Part model, mm, in its own coordinate system. Face numbers are marked on the shaded views. A direction names the side the tool comes from. Round coordinates to 2 decimals unless told otherwise and drop trailing zeros. Write each loop counter-clockwise with the first axis right and the second up, starting at its lowest first coordinate (ties: lowest second). Pieces come first, ordered by that corner, then holes. Notation, with made-up numbers: M 74.25,-10 L 92.25,-10 A17 ccw 92.25,1 Z; hole C 4.5,-11 d10. An arc over 180 degrees is marked long. Answer as a JSON object with one key per item and string values. Group by question number.
1. Which spindle directions (+Z, -Z, +X, -X, +Y, -Y) get a long thin tool onto all of the face, cutting with end or side? Do the marked faces 1, 2 and 3. Say none if no direction does.
2. Drill centre lines: line 1 (Z direction, x = 0, y = 3.6); line 2 (Z direction, x = -4.5, y = 2.45); line 3 (X direction, y = 2.7, z = 0). Where is each one in solid material? Low to high. Write a range as from..to.
3. Drop a flat-ended pin along its axis: pin 1 (1.5 mm diameter, centred on x = -4, y = 1, fed in from +Z). Give the stop position or say it passes through.
4. Band-saw the part on C-C, the plane z = -4.25. Write the cut outline in (x, y).
5. Band-saw the part on A-A, the plane z = 0. Write the cut outline in (x, y), plus the area to 3 significant figures.
6. Two-plate mould, pull along X, no slides. Class the marked faces 4, 5 and 6: +X half, -X half, draft (parallel to the pull), parting line (faces both ways), or undercut.
7. Band-saw the part on B-B, the plane x = 0. Write the cut outline in (y, z).
Autodesk Inventor part; units mm, degrees
ref_plane "YZ Plane" through (0, 0, 0) normal (1, 0, 0) x (0, 1, 0)
ref_plane "XZ Plane" through (0, 0, 0) normal (0, 1, 0) x (-1, 0, 0)
ref_plane "XY Plane" through (0, 0, 0) normal (0, 0, 1) x (1, 0, 0)
sketch "Sketch1" plane through (0, 0, 0) normal (0, 1, 0) x (-1, 0, 0)
  arc A0 (0.45, -5.5819) -> (-0.45, -5.5819) centre (0, 0) ccw construction
  circle A1 centre (0, 0) radius 4.15
  line L0 (-0.45, -5.5819) -> (-0.675, -4.0947)
  line L1 (0.675, -4.0947) -> (0.45, -5.5819)
  line L2 (0.675, -4.0947) -> (-0.675, -4.0947) construction
  line L3 (0.45, -5.5819) -> (-0.45, -5.5819) construction
  arc A2 (-0.45, -5.5819) -> (0.45, -5.5819) centre (0, 0) ccw
  circle A3 centre (0, 0) radius 3 construction
  circle A4 centre (0, 0) radius 3.15
  line L4 (2.7807, 1.48) -> (-2.7807, 1.48)
  dimension "d1" = 11.2
  dimension "d2" = 8.3
  dimension "d3" = 0.9
  dimension "d4" = 1.35
  dimension "d13" = 6
  dimension "d16" = 0.15
  dimension "d17" = 1.48
extrude "Extrusion1" add sketch "Sketch1" along normal blind 4 contours A1 | A4 L4 | L4 A4
extrude "Extrusion2" add sketch "Sketch1" along normal blind 4 contours A1 L1 A2 L0
fillet "Fillet1" radius 0.3 2 edges at (0.45, 2, -5.5819) (-0.45, 2, -5.5819)
pattern_circular "Circular Pattern1" count 12 over 360 about axis through (0, 0, 0) along (0, 1, 0) of "Extrusion2", "Fillet1"
extrude "Extrusion3" cut sketch "Sketch1" along normal blind 4 contours A4 L4 picked at (1.2217, -1.3888)
properties part number "Motor Shaft Gear E" material "ABS Plastic"
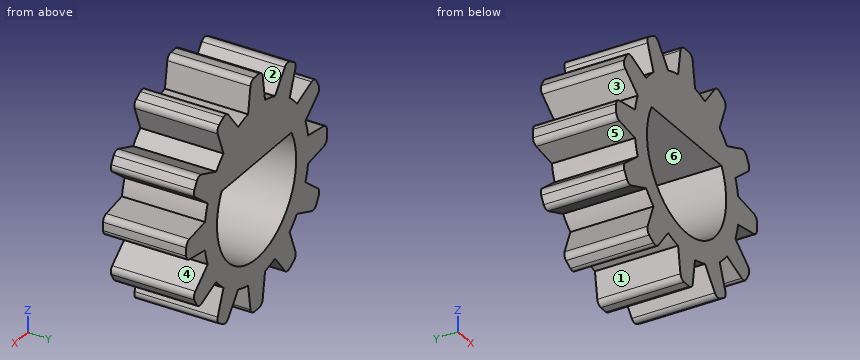
Worked answers:
{
 "1": {"face 1": "-Z, +Y, -Y", "face 2": "+Z, +Y, -Y", "face 3": "-X, +Y, -Y"},
 "2": {"line 1": "z = -5.6..-3.15, 1.48..5.6", "line 2": "z = -3.11..-1.95, -0.61..0.61, 1.95..3.11", "line 3": "x = -5.6..-3.15, 3.15..5.6"},
 "3": {"pin 1": "stops at z = 3.11"},
 "4": {"outline": "M -3.04,0 L -1.76,0 L -1.76,4 L -3.04,4 Z; M -0.65,0 L 0.65,0 L 0.65,4 L -0.65,4 Z; M 1.76,0 L 3.04,0 L 3.04,4 L 1.76,4 Z"},
 "5": {"outline": "M -5.6,0 L -3.15,0 L -3.15,4 L -5.6,4 Z; M 3.15,0 L 5.6,0 L 5.6,4 L 3.15,4 Z", "area": "19.6 mm^2"},
 "6": {"face 4": "+X half", "face 5": "-X half", "face 6": "undercut"},
 "7": {"outline": "M 0,-5.6 L 4,-5.6 L 4,-3.15 L 0,-3.15 Z; M 0,1.48 L 4,1.48 L 4,5.6 L 0,5.6 Z"}
}
